Geometry: see drawing. Coordinates: mm, zero at the bounding-box minimum. Give positions to 0.01 mm unless a question says otherwise; leave off trailing zeros. Order: outer loops, then holes, each group sorted by start corner. A loop starts at its lowest first (then second) coordinate and runs counter-clockwise, first axis right, second up. Notation, with made-up numbers: (63, 64.25) - (84, 64.25) arc R13 cw to (84, 72.25) - close; hole circle Ø11 at (78.25, 42). An arc over 180 degrees is marked (long way). Write each question's results on one line, items separated by ' | '. Start each with the question number.
Item 1: Contact query for flat-ended pins moving along their axis: pin 1 Ø4.5 at (x, z) = (37.5, 70) entering from +Y; pin 2 Ø8 at (x, y) = (22, 9.5) entering from -Z; pin 3 Ø8 at (x, y) = (33, 6.5) entering from -Z. Output: stop coordinate, or through.
Item 2: Section C-C on x = 70. Output: boundary loops of the cut face in (y, z).
Item 3: Section A-A on z = 37.5. Output: boundary loops of the cut face in (x, y).
Item 4: Mould query, pull axis X, two halves, no side actions, for the marked faces 1, 2 and 3. Classes: released by +X, released by -X, zero draft, split by the parting line, or undercut.
Item 5: Section D-D on y = 11.75. Output: boundary loops of the cut face in (x, z).
Item 6: Section B-B on z = 70. Output: boundary loops of the cut face in (x, y).
Item 7: Line query: line 1 along X through (y, z) = (5.5, 37.5); line 2 along Y through (x, z) = (67, 23.5); line 3 along Z through (x, y) = (70, 3). Output: solid intervals per line, ascending.
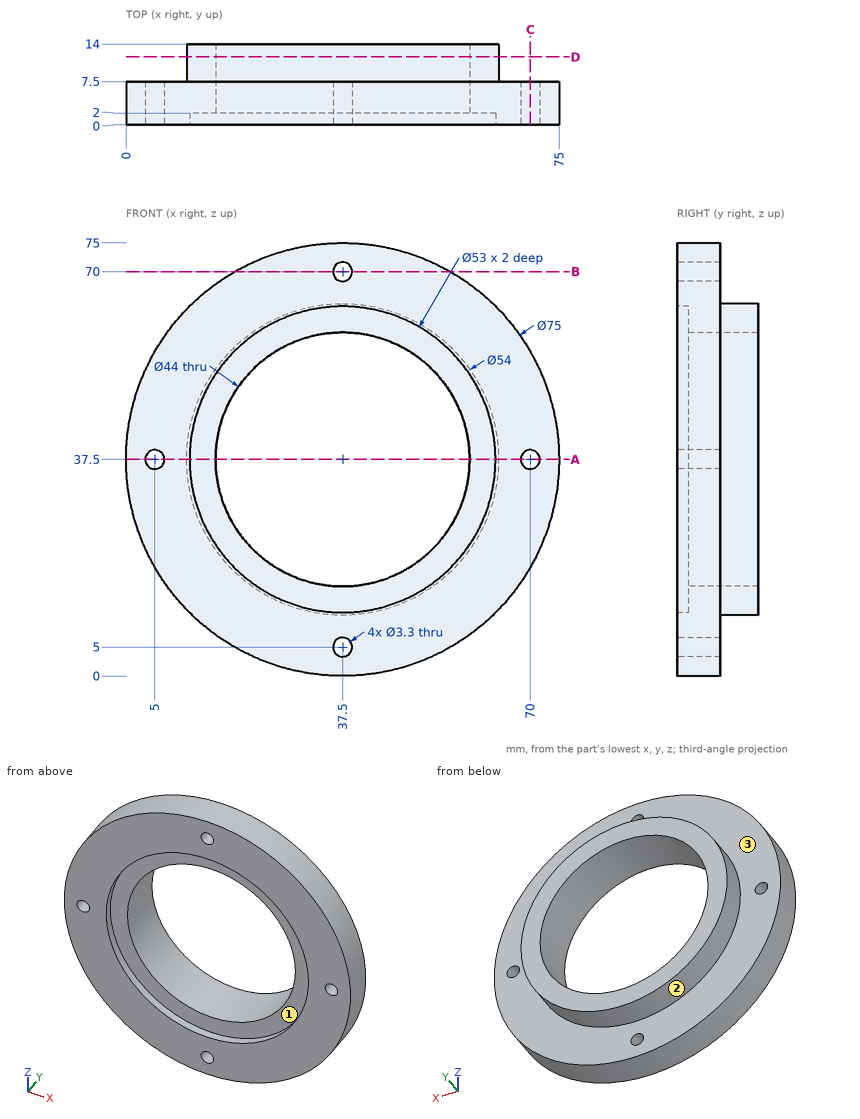
Evaluation:
1) pin 1: stops at y = 7.5 | pin 2: stops at z = 1.98 | pin 3: stops at z = 0
2) outline: (0, 18.79) - (7.5, 18.79) - (7.5, 35.85) - (0, 35.85) - close; (0, 39.15) - (7.5, 39.15) - (7.5, 56.21) - (0, 56.21) - close
3) outline: (0, 0) - (3.35, 0) - (3.35, 7.5) - (0, 7.5) - close; (6.65, 0) - (11, 0) - (11, 2) - (15.5, 2) - (15.5, 14) - (10.5, 14) - (10.5, 7.5) - (6.65, 7.5) - close; (59.5, 2) - (64, 2) - (64, 0) - (68.35, 0) - (68.35, 7.5) - (64.5, 7.5) - (64.5, 14) - (59.5, 14) - close; (71.65, 0) - (75, 0) - (75, 7.5) - (71.65, 7.5) - close
4) face 1: undercut | face 2: split by the parting line | face 3: zero draft
5) outline: circle Ø54 at (37.5, 37.5); hole circle Ø44 at (37.5, 37.5)
6) outline: (18.79, 0) - (35.85, 0) - (35.85, 7.5) - (18.79, 7.5) - close; (39.15, 0) - (56.21, 0) - (56.21, 7.5) - (39.15, 7.5) - close
7) line 1: x = 0 to 3.35, 6.65 to 15.5, 59.5 to 68.35, 71.65 to 75 | line 2: y = 0 to 7.5 | line 3: z = 18.79 to 35.85, 39.15 to 56.21
